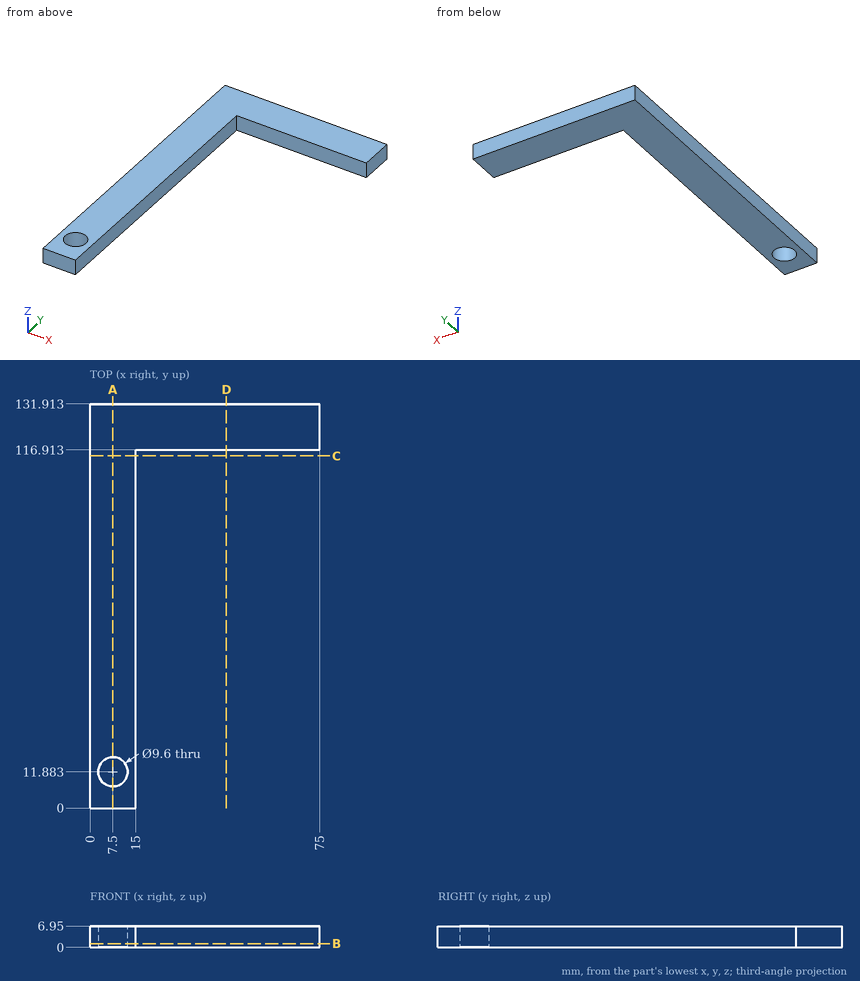
Here's the drawing with two shaded views (mm, measured from the low corner). I have some questions. Coordinates: 2 decimals unless noted, no trailing zeros. Write each loop counter-clockwise with the first axis right and the second up, starting at its lowest first coordinate (ties: lowest second). Pieces come first, ordered by that corner, then holes.
Item 1: I want a section at C-C on y = 115. Write out the boundary of the cut face in (x, z), and give its area (3 significant figures).
Item 2: Will these pins go through, and if not, where does the flat tip stop? pin 1 (1 mm diameter, centred on x = 61, z = 6, fed in from -Y); pin 2 (10 mm diameter, centred on x = 11.5, y = 60, fed in from -Z).
Item 3: I want a section at D-D on x = 44.5. Write out the boundary of the cut face in (y, z).
Item 4: If I drill on line 1 (Y direction, x = 7.5, z = 4.5); line 2 (Y direction, x = 25, z = 4); line 3 (X direction, y = 58, z = 3), over which ranges is the centre line in solid material (lowest first)?
Item 5: I want a section at A-A on x = 7.5. Write out the boundary of the cut face in (y, z).
Item 6: I want a section at B-B on z = 1.25. Write out the boundary of the cut face in (x, y), and give its area (3 significant figures).
Findings below:
1. outline: (0, 0) - (15, 0) - (15, 6.95) - (0, 6.95) - close
1. area: 104 mm2
2. pin 1: stops at y = 116.91
2. pin 2: stops at z = 0
3. outline: (116.91, 0) - (131.91, 0) - (131.91, 6.95) - (116.91, 6.95) - close
4. line 1: y = 0 to 7.08, 16.68 to 131.91
4. line 2: y = 116.91 to 131.91
4. line 3: x = 0 to 15
5. outline: (0, 0) - (7.08, 0) - (7.08, 6.95) - (0, 6.95) - close; (16.68, 0) - (131.91, 0) - (131.91, 6.95) - (16.68, 6.95) - close
6. outline: (0, 0) - (15, 0) - (15, 116.91) - (75, 116.91) - (75, 131.91) - (0, 131.91) - close; hole circle Ø9.6 at (7.5, 11.88)
6. area: 2,810 mm2
